```python
from build123d import *

# Parameters (mm, degrees)
CROQUIS1_R              = 1.58
SALIENTE_EXTRUIR1_DEPTH = 4


with BuildPart() as part:
    # Croquis1 → Saliente-Extruir1 (new body)
    with BuildSketch(Plane.XY):
        with BuildLine():
            Line((26.538050923, 6.699416954), (53.838050923, 6.699416954))
            ThreePointArc((53.838050923, 6.699416954), (58.328178983, 4.839545014), (60.188050923, 0.349416954))
            Line((60.188050923, 0.349416954), (60.188050923, -17.045643676))
            ThreePointArc((60.188050923, -17.045643676), (62.047922862, -21.535771736), (66.538050923, -23.395643676))
            Line((66.538050923, -23.395643676), (73.838050923, -23.395643676))
            ThreePointArc((73.838050923, -23.395643676), (78.328178983, -21.535771736), (80.188050923, -17.045643676))
            Line((80.188050923, -17.045643676), (80.188050923, 6.604356324))
            Line((80.188050923, 6.604356324), (80.188050923, 20.254356324))
            ThreePointArc((80.188050923, 20.254356324), (78.328178983, 24.744484385), (73.838050923, 26.604356324))
            Line((73.838050923, 26.604356324), (6.538050923, 26.604356324))
            ThreePointArc((6.538050923, 26.604356324), (2.047922862, 24.744484385), (0.188050923, 20.254356324))
            Line((0.188050923, 20.254356324), (0.188050923, 6.604356324))
            Line((0.188050923, 6.604356324), (0.188050923, -17.045643676))
            ThreePointArc((0.188050923, -17.045643676), (2.047922862, -21.535771736), (6.538050923, -23.395643676))
            Line((6.538050923, -23.395643676), (13.838050923, -23.395643676))
            ThreePointArc((13.838050923, -23.395643676), (18.328178983, -21.535771736), (20.188050923, -17.045643676))
            Line((20.188050923, -17.045643676), (20.188050923, 0.349416954))
            ThreePointArc((20.188050923, 0.349416954), (22.047922862, 4.839545014), (26.538050923, 6.699416954))
        make_face()
        with Locations((40.188050923, 15.866498333)):
            Circle(CROQUIS1_R, mode=Mode.SUBTRACT)
        with Locations((10.188050923, 15.866498333)):
            Circle(CROQUIS1_R, mode=Mode.SUBTRACT)
        with Locations((70.188050923, 15.771437703)):
            Circle(CROQUIS1_R, mode=Mode.SUBTRACT)
        with Locations((10.188050923, -5.676497666)):
            Circle(CROQUIS1_R, mode=Mode.SUBTRACT)
        with Locations((70.188050923, -5.771558296)):
            Circle(CROQUIS1_R, mode=Mode.SUBTRACT)
    extrude(amount=SALIENTE_EXTRUIR1_DEPTH)


solid = part.part
```
Read the model definition and answer for the solid it produces. Units are mm, in the model's axes. A direction names the side the tool comes from. Give positions to 0.01 mm unless a question says otherwise; leave off trailing zeros. Order: outer loops, then holes, each group sorted by start corner. A loop starts at its lowest first (then second) coordinate and runs counter-clockwise, first axis right, second up.
(1) For a pull along Y with two mould halves and no side action, classify faces 3 (the cylindrical face through (78.38, 24.69, 1.97)), 4 (the flat face through (0.188, 2, 2)), 5 (the cylindrical face through (41.648, 15.261, 1.972)) as released by +Y, released by -Y, zero draft, split by the parting line, or undercut.
(2) Find section A-A (y = 1.5). Give the vertices of the cut face in (x, z).
(3) Straight lines are drawn through the part: L1, parallel to X at y = 16, z = 1.45; L2, parallel to X at y = -17.5, z = 0.65; L3, parallel to X at y = -6, z = 1.25. For each, find the intervals that lie inside material, in ascending order.
(4) Find section B-B (x = 41). Give the vertices of the cut face in (y, z).
(5) Find section D-D (x = 25). Give the vertices of the cut face in (y, z).
(6) Given pin 1 (3.5 mm diameter, centred on x = 40.19, y = 15.87, fed in from -Z); pin 2 (1.2 mm diameter, centred on x = 39.5, z = 2, fed in from -Y); pin 3 (3 mm diameter, centred on x = 10.19, y = 15.87, fed in from -Z), each flat-ended and moving along its own axis, determine where each tip first touches the part or whether it passes through.
(7) Find section C-C (z = 1.55). Give the vertices of the cut face in (x, y), plus the area to 3 significant figures.
(8) For faces 1 (the cylindrical face through (18.279, -21.585, 1.972)), 2 (the cylindrical face through (2.098, 24.794, 1.972)), determine the directions among +Z, -Z, +X, -X, +Y, -Y from which every point of the face is accessible in a straight line to the end or side of a thin tool.
Result sheet:
1. face 3: released by +Y
1. face 4: zero draft
1. face 5: undercut
2. outline: (0.19, 0) - (20.29, 0) - (20.29, 4) - (0.19, 4) - close; (60.08, 0) - (80.19, 0) - (80.19, 4) - (60.08, 4) - close
3. L1: x = 0.19 to 8.61, 11.76 to 38.61, 41.76 to 68.62, 71.75 to 80.19
3. L2: x = 0.2 to 20.17, 60.2 to 80.17
3. L3: x = 0.19 to 8.64, 11.73 to 20.19, 60.19 to 68.62, 71.75 to 80.19
4. outline: (6.7, 0) - (14.51, 0) - (14.51, 4) - (6.7, 4) - close; (17.22, 0) - (26.6, 0) - (26.6, 4) - (17.22, 4) - close
5. outline: (6.51, 0) - (26.6, 0) - (26.6, 4) - (6.51, 4) - close
6. pin 1: stops at z = 0
6. pin 2: stops at y = 6.7
6. pin 3: passes through
7. outline: (0.19, -17.05) arc R6.35 ccw to (6.54, -23.4) - (13.84, -23.4) arc R6.35 ccw to (20.19, -17.05) - (20.19, 0.35) arc R6.35 cw to (26.54, 6.7) - (53.84, 6.7) arc R6.35 cw to (60.19, 0.35) - (60.19, -17.05) arc R6.35 ccw to (66.54, -23.4) - (73.84, -23.4) arc R6.35 ccw to (80.19, -17.05) - (80.19, 20.25) arc R6.35 ccw to (73.84, 26.6) - (6.54, 26.6) arc R6.35 ccw to (0.19, 20.25) - close; hole circle Ø3.16 at (10.19, -5.68); hole circle Ø3.16 at (10.19, 15.87); hole circle Ø3.16 at (40.19, 15.87); hole circle Ø3.16 at (70.19, -5.77); hole circle Ø3.16 at (70.19, 15.77)
7. area: 2,720 mm2
8. face 1: +Z, -Z, -Y
8. face 2: +Z, -Z, -X, +Y
